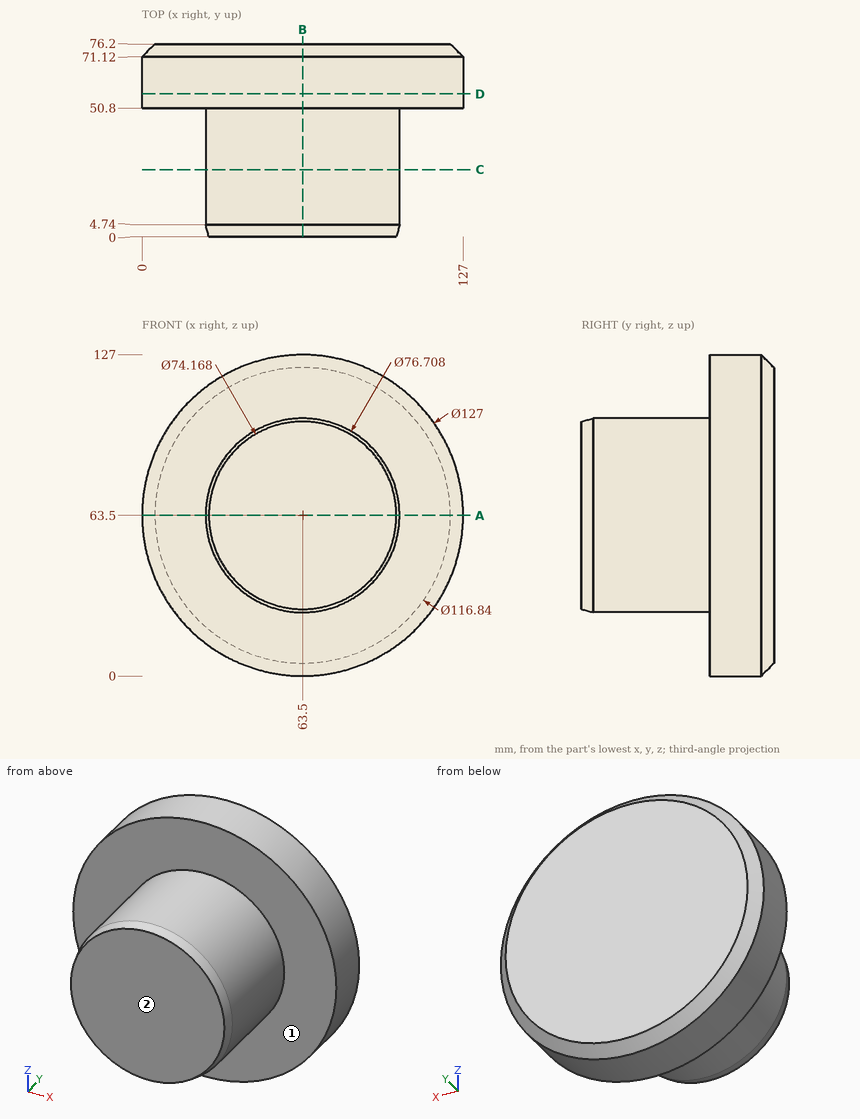
Study the drawing (mm; zero at the part's minimum x, y, z) and answer. A direction names the side the tool comes from. Coordinates: 2 decimals unless noted, no trailing zeros. Loops run counter-clockwise (first coordinate to the right, second up) from the corner with the lowest first, then second, coordinate; pieces in that order, holes last. Notation, with made-up numbers: M 79.5,-14.75 L 88.5,-14.75 A25 ccw 88.5,12.25 Z; hole C -5,48 d2. An arc over 180 degrees is marked long. Answer as a JSON object with one key per item and string values. Group by question number.
Item 1: Section A-A (z = 63.5) is taken. Write down the section's boundary in (x, y).
Item 2: Each of these flat-tipped pins is pushed along its axis until it touches: P1, Ø12, axis at y = 15, z = 27, coming from the -X side (1 decimal); P2, Ø3, axis at x = 28, y = 32.5, coming from the +Z side; P3, Ø12, axis at x = 78.5, y = 50, coming from the +Z side. Where does it stop, or does it pass through?
Item 3: Which of the six approach directions +Z, -Z, +X, -X, +Y, -Y give full straight-line access (tool end or side, diameter ignored) to the marked faces 1 and 2?
Item 4: Section C-C (y = 26.5) is taken. Write down the section's boundary in (x, z), and give its area (3 significant figures).
Item 5: Section B-B (x = 63.5) is taken. Write down the section's boundary in (y, z), and give its area (3 significant figures).
Item 6: Consider L1, parallel to Y at x = 63, z = 110; L2, parallel to Z at x = 62.5, y = 42; L3, parallel to Z at x = 75, y = 68. Determine where each line is inside the solid, lowest interval first.
Item 7: Section D-D (y = 56.5) is taken. Write down the section's boundary in (x, z), and give its area (3 significant figures).
Solved:
{
 "1": {"outline": "M 0,50.8 L 25.15,50.8 L 25.15,4.74 L 26.42,0 L 100.58,0 L 101.85,4.74 L 101.85,50.8 L 127,50.8 L 127,71.12 L 121.92,76.2 L 5.08,76.2 L 0,71.12 Z"},
 "2": {"P1": "stops at x = 40.2", "P2": "stops at z = 81.25", "P3": "stops at z = 126.35"},
 "3": {"face 1": "-Y", "face 2": "+Z, -Z, +X, -X, -Y"},
 "4": {"outline": "C 63.5,63.5 d76.71", "area": "4,620 mm2"},
 "5": {"outline": "M 0,26.42 L 4.74,25.15 L 50.8,25.15 L 50.8,0 L 71.12,0 L 76.2,5.08 L 76.2,121.92 L 71.12,127 L 50.8,127 L 50.8,101.85 L 4.74,101.85 L 0,100.58 Z", "area": "7,090 mm2"},
 "6": {"L1": "y = 50.8 to 76.2", "L2": "z = 25.16 to 101.84", "L3": "z = 1.05 to 125.95"},
 "7": {"outline": "C 63.5,63.5 d127", "area": "12,700 mm2"}
}
